Source: CAD feature listing. Evaluate the final solid. Frame: model axes, mm. A direction names the side the tool comes from. Give positions to 0.01 mm unless a question says otherwise; leave off trailing zeros. Write each loop counter-clockwise with the first axis right and the second up, starting at its lowest first coordinate (ties: lowest second). Pieces come first, ordered by that corner, then holes. Notation, with made-up numbers: (85.25, 24.5) -> (125.25, 24.5) arc R29 cw to (125.25, 55.5) -> close; hole circle Ø9 at (-27.5, -8). An arc over 180 degrees is marked (long way). Write item = value, one per line.
from build123d import *

# Parameters (mm, degrees)
SKETCH1_R           = 2.5
BOSS_EXTRUDE1_DEPTH = 10
FILLET1_R           = 25
FILLET2_R           = 2


with BuildPart() as part:
    # Sketch1 → Boss-Extrude1 (new body)
    with BuildSketch(Plane(origin=(0, 0, 0), x_dir=(1, 0, 0), z_dir=(0, 1, 0))):
        with BuildLine():
            Line((0, 0), (-300, 0))
            Line((-300, 0), (-300, 125))
            Line((-300, 125), (-287.5, 155))
            Line((-287.5, 155), (-275, 125))
            Line((-275, 125), (-275, 107))
            Line((-275, 107), (-292.60586559, 63.771946566))
            ThreePointArc((-292.60586559, 63.771946566), (-285.266321562, 50.186402284), (-273.344525562, 60))
            Line((-273.344525562, 60), (-273.344525562, 84))
            ThreePointArc((-273.344525562, 84), (-266.980564532, 81.363961031), (-264.344525562, 75))
            Line((-264.344525562, 75), (-264.344525562, 25))
            Line((-264.344525562, 25), (-255.344525562, 25))
            Line((-255.344525562, 25), (-255.344525563, 77))
            Line((-255.344525563, 77), (-263.518505835, 94))
            ThreePointArc((-263.518505835, 94), (-264.580199309, 104.023888208), (-259.057764575, 112.456458543))
            Line((-259.057764575, 112.456458543), (-242.5, 125))
            Line((-242.5, 125), (-230, 155))
            Line((-230, 155), (-217.5, 125))
            Line((-217.5, 125), (-217.5, 107))
            Line((-217.5, 107), (-235.10586559, 63.771946566))
            ThreePointArc((-235.10586559, 63.771946566), (-227.766321562, 50.186402284), (-215.844525562, 60))
            Line((-215.844525562, 60), (-215.844525562, 84))
            ThreePointArc((-215.844525562, 84), (-209.480564532, 81.363961031), (-206.844525562, 75))
            Line((-206.844525562, 75), (-206.844525562, 25))
            Line((-206.844525562, 25), (-197.844525562, 25))
            Line((-197.844525562, 25), (-197.844525563, 77))
            Line((-197.844525563, 77), (-206.018505835, 94))
            ThreePointArc((-206.018505835, 94), (-207.080199309, 104.023888208), (-201.557764575, 112.456458543))
            Line((-201.557764575, 112.456458543), (-185, 125))
            Line((-185, 125), (-172.5, 155))
            Line((-172.5, 155), (-160, 125))
            Line((-160, 125), (-160, 107))
            Line((-160, 107), (-177.60586559, 63.771946566))
            ThreePointArc((-177.60586559, 63.771946566), (-170.266321562, 50.186402284), (-158.344525563, 60))
            Line((-158.344525563, 60), (-158.344525563, 84))
            ThreePointArc((-158.344525563, 84), (-151.980564532, 81.363961031), (-149.344525563, 75))
            Line((-149.344525563, 75), (-149.344525563, 25))
            Line((-149.344525563, 25), (-140.344525563, 25))
            Line((-140.344525563, 25), (-140.344525563, 77))
            Line((-140.344525563, 77), (-148.518505835, 94))
            ThreePointArc((-148.518505835, 94), (-149.580199309, 104.023888208), (-144.057764575, 112.456458543))
            Line((-144.057764575, 112.456458543), (-127.5, 125))
            Line((-127.5, 125), (-115, 155))
            Line((-115, 155), (-102.5, 125))
            Line((-102.5, 125), (-102.5, 107))
            Line((-102.5, 107), (-120.10586559, 63.771946566))
            ThreePointArc((-120.10586559, 63.771946566), (-112.766321562, 50.186402284), (-100.844525563, 60))
            Line((-100.844525563, 60), (-100.844525563, 84))
            ThreePointArc((-100.844525563, 84), (-94.480564532, 81.363961031), (-91.844525563, 75))
            Line((-91.844525563, 75), (-91.844525563, 25))
            Line((-91.844525563, 25), (-82.844525563, 25))
            Line((-82.844525563, 25), (-82.844525563, 77))
            Line((-82.844525563, 77), (-91.018505835, 94))
            ThreePointArc((-91.018505835, 94), (-92.080199309, 104.023888208), (-86.557764575, 112.456458543))
            Line((-86.557764575, 112.456458543), (-70, 125))
            Line((-70, 125), (-57.5, 155))
            Line((-57.5, 155), (-45, 125))
            Line((-45, 125), (-45, 107))
            Line((-45, 107), (-62.60586559, 63.771946566))
            ThreePointArc((-62.60586559, 63.771946566), (-55.266321562, 50.186402284), (-43.344525562, 60))
            Line((-43.344525562, 60), (-43.344525562, 84))
            ThreePointArc((-43.344525562, 84), (-36.980564532, 81.363961031), (-34.344525562, 75))
            Line((-34.344525562, 75), (-34.344525562, 25))
            Line((-34.344525562, 25), (-25.344525562, 25))
            Line((-25.344525562, 25), (-25.344525563, 77))
            Line((-25.344525563, 77), (-33.518505835, 94))
            ThreePointArc((-33.518505835, 94), (-34.580199309, 104.023888208), (-29.057764575, 112.456458543))
            Line((-29.057764575, 112.456458543), (-12.5, 125))
            Line((-12.5, 125), (0, 155))
            Line((0, 155), (0, 0))
        make_face()
        with Locations(Location((-5, 125, 0), (0, 0, 270))):
            Circle(SKETCH1_R, mode=Mode.SUBTRACT)
        with Locations(Location((-61.5, 89, 0), (0, 0, 270))):
            Circle(SKETCH1_R, mode=Mode.SUBTRACT)
        with Locations(Location((-62.5, 125, 0), (0, 0, 270))):
            Circle(SKETCH1_R, mode=Mode.SUBTRACT)
        with Locations(Location((-119, 89, 0), (0, 0, 270))):
            Circle(SKETCH1_R, mode=Mode.SUBTRACT)
        with Locations(Location((-120, 125, 0), (0, 0, 270))):
            Circle(SKETCH1_R, mode=Mode.SUBTRACT)
        with Locations(Location((-176.5, 89, 0), (0, 0, 270))):
            Circle(SKETCH1_R, mode=Mode.SUBTRACT)
        with Locations(Location((-177.5, 125, 0), (0, 0, 270))):
            Circle(SKETCH1_R, mode=Mode.SUBTRACT)
        with Locations(Location((-234, 89, 0), (0, 0, 270))):
            Circle(SKETCH1_R, mode=Mode.SUBTRACT)
        with Locations(Location((-235, 125, 0), (0, 0, 270))):
            Circle(SKETCH1_R, mode=Mode.SUBTRACT)
        with Locations(Location((-291.5, 89, 0), (0, 0, 270))):
            Circle(SKETCH1_R, mode=Mode.SUBTRACT)
    extrude(amount=BOSS_EXTRUDE1_DEPTH)

    # Fillet1
    fillet1_edges = [part.edges().sort_by_distance(p)[0] for p in [
        (-275, 5, -125),
        (-275, 5, -107),
        (-255.344525563, 5, -77),
        (-242.5, 5, -125),
        (-217.5, 5, -125),
        (-217.5, 5, -107),
        (-197.844525563, 5, -77),
        (-185, 5, -125),
        (-160, 5, -125),
        (-160, 5, -107),
        (-140.344525563, 5, -77),
        (-127.5, 5, -125),
        (-102.5, 5, -125),
        (-102.5, 5, -107),
        (-82.844525563, 5, -77),
        (-70, 5, -125),
        (-45, 5, -125),
        (-45, 5, -107),
        (-25.344525563, 5, -77),
        (-12.5, 5, -125),
    ]]
    fillet(fillet1_edges, radius=FILLET1_R)

    # Fillet2
    fillet2_edges = [part.edges().sort_by_distance(p)[0] for p in [
        (-273.344525562, 5, -84),
        (-215.844525562, 5, -84),
        (-158.344525563, 5, -84),
        (-100.844525563, 5, -84),
        (-43.344525562, 5, -84),
    ]]
    fillet(fillet2_edges, radius=FILLET2_R)


solid = part.part
(1) Section query A-A (z = -30). Return loops of the section in (x, y).
Values follow:
outline = (-300, 0) -> (-264.34, 0) -> (-264.34, 10) -> (-300, 10) -> close; (-255.34, 0) -> (-206.84, 0) -> (-206.84, 10) -> (-255.34, 10) -> close; (-197.84, 0) -> (-149.34, 0) -> (-149.34, 10) -> (-197.84, 10) -> close; (-140.34, 0) -> (-91.84, 0) -> (-91.84, 10) -> (-140.34, 10) -> close; (-82.84, 0) -> (-34.34, 0) -> (-34.34, 10) -> (-82.84, 10) -> close; (-25.34, 0) -> (0, 0) -> (0, 10) -> (-25.34, 10) -> close
(2) Material intervals for line 1 (X direction, y = 2.25, z = -47.5); line 2 (X direction, y = 7.75, z = -101.5); line 3 (Z direction, x = -176.5, y = 4.75), sorted ascending.
Values follow:
line_1 = -300 to -264.34, -255.34 to -206.84, -197.84 to -149.34, -140.34 to -91.84, -82.84 to -34.34, -25.34 to 0
line_2 = -300 to -277.24, -264.97 to -219.74, -207.47 to -162.24, -149.97 to -104.74, -92.47 to -47.24, -34.97 to 0
line_3 = -145.4 to -127.29, -122.71 to -91.5, -86.5 to -66.49, -54.21 to 0
(3) Section query B-B (y = 6). Give the number of separate pieces and of enclosed holes in the cut face, plus the area to 3 significant figures.
Values follow:
separate_pieces = 1
enclosed_holes = 10
area = 30,200 mm2
(4) Pull-direction query (X, two-part tool) for faces 1 (the face through (-255.345, 5, -48)), 2 (the face through (-148, 10, -96)); classes: pulls with the +X half, pulls with the -X half, needs draft (parallel to the pull), parting line crosses it, or undercut.
Values follow:
face_1 = undercut
face_2 = needs draft
(5) First-contact query: pin 1 (2.5 mm diameter, centred on x = -203.5, y = 5.5, fed in from -Z); pin 2 (1.5 mm diameter, centred on x = -184.5, y = 6, fed in from -Z); pin 3 (2.5 mm diameter, centred on x = -30.5, y = 4, fed in from -Z). Flat tips, straight axial feed; report the tip coordinate or a pass-through.
Values follow:
pin_1 = -111.9
pin_2 = -128.49
pin_3 = -112.31
(6) Access query for faces 3 (the face through (-145, 5, -25)), 4 (the face through (-100.845, 5, -71)). Directions: +Z, -Z, +X, -X, +Y, -Y. A direction counts if a zero-diameter tool reaches every point of the face in a straight line with its end or side. Return the directions, or none.
Values follow:
face_3 = +Y, -Y
face_4 = -Z, +Y, -Y
